Here's how the part is built. I have some questions about the finished solid (model axes, mm). A direction names the side the tool comes from. Give positions to 0.01 mm unless a question says otherwise; leave off trailing zeros. Loops run counter-clockwise (first coordinate to the right, second up) from the corner with the lowest first, then second, coordinate; pieces in that order, holes last.
Q1. Will these pins go through, and if not, where does the flat tip stop? P1, Ø8.5, axis at x = 6, y = -1, coming from the +Z side; P2, Ø24, axis at x = -3.5, y = 3, coming from the +Z side; P3, Ø6, axis at x = 0, y = 0, coming from the +Z side; P4, Ø1.2, axis at x = 0, y = 17, coming from the +Z side.
Q2. For faces 4 (the face through (0, -20, 2)), 5 (the face through (0, 24, 5)), which set-ups out of +Z, -Z, +X, -X, +Y, -Y let a thin tool reach every point of the face, with its end or its side?
Q3. If we section it at C-C (z = -2): Please give me the cut outline in (x, y), plus the area to 3 significant figures.
Q4. If we section it at D-D (y = -9.5): Please give me the cut outline in (x, z), plus the area to 3 significant figures.
Q5. We'd pull the mould along Z, two halves only. Please class faces 1 (the face through (0, 8, -5)), 2 (the face through (0, -6, 7)), 3 (the face through (0, 25, 2)): +Z half, -Z half, draft (parallel to the pull), parting line (faces both ways), or undercut.
Q6. I need wall thicknesses on line 1 (X direction, y = 0, z = 7.35); line 2 (Y direction, x = 0, z = 2.5); line 3 (Y direction, x = 0, z = 7.15). Which ranges of each line are inside material? Lowest first, please.
Q7. If we section it at B-B (z = 3.25): Give the number of separate pieces and of enclosed holes in the cut face, plus the area to 3 significant figures.
Q8. If we section it at A-A (y = 0): Please give me the cut outline in (x, z), plus the area to 3 significant figures.
from build123d import *

# Parameters (mm, degrees)
SKETCH_R          = 15
PAD_DEPTH         = 7
SKETCH001_R       = 2
PAD001_DEPTH      = 5
SKETCH002_R       = 15
SKETCH002_R_2     = 14
PAD002_DEPTH      = 7.4
SKETCH003_W       = 50
SKETCH003_H       = 45
PAD003_DEPTH      = 5
SKETCH004_W       = 50
SKETCH004_H       = 45
SKETCH004_W_2     = 48
SKETCH004_H_2     = 43
PAD004_DEPTH      = 10
SKETCH005_R       = 5
POCKET_DEPTH      = 5.001
POCKET_DEPTH_BACK = -10.001
SKETCH006_R       = 2
POCKET001_DEPTH   = 4


with BuildPart() as part:
    # Sketch → Pad (new body)
    with BuildSketch(Plane.XY):
        Circle(SKETCH_R)
    extrude(amount=PAD_DEPTH)

    # Sketch001 → Pad001 (join)
    with BuildSketch(Plane.XY):
        with BuildLine():
            add(Edge.make_bspline(
                [(-9.089263, 11.932531), (-7.058013, 18.679317), (0, 23.549677), (7.058013, 18.679317), (9.089263, 11.932531)],
                knots=[0, 0, 0, 0, 0.5, 1, 1, 1, 1], degree=3))
            Line((9.089263, 11.932531), (-9.089263, 11.932531))
        make_face()
        with Locations((0, 17.442505)):
            Circle(SKETCH001_R, mode=Mode.SUBTRACT)
    extrude(amount=PAD001_DEPTH)

    # Sketch002 → Pad002 (join)
    with BuildSketch(Plane.XY):
        Circle(SKETCH002_R)
        Circle(SKETCH002_R_2, mode=Mode.SUBTRACT)
    extrude(amount=PAD002_DEPTH)

    # Sketch003 → Pad003 (join)
    with BuildSketch(Plane.XY):
        with Locations((0, 2.5)):
            Rectangle(SKETCH003_W, SKETCH003_H)
    extrude(amount=-PAD003_DEPTH)

    # Sketch004 → Pad004 (join)
    with BuildSketch(Plane.XY):
        with Locations((0, 2.5)):
            Rectangle(SKETCH004_W, SKETCH004_H)
        with Locations((0, 2.5)):
            Rectangle(SKETCH004_W_2, SKETCH004_H_2, mode=Mode.SUBTRACT)
    extrude(amount=PAD004_DEPTH)

    # Sketch005 → Pocket (cut, two sides)
    with BuildSketch(Plane.XY) as pocket_sk:
        Circle(SKETCH005_R)
    extrude(amount=-POCKET_DEPTH, mode=Mode.SUBTRACT)
    extrude(pocket_sk.sketch, amount=-POCKET_DEPTH_BACK, mode=Mode.SUBTRACT)

    # Sketch006 → Pocket001 (cut)
    with BuildSketch(Plane.XY):
        with Locations((0, 17.442505)):
            Circle(SKETCH006_R)
    extrude(amount=-POCKET001_DEPTH, mode=Mode.SUBTRACT)


solid = part.part
Check sheet entries:
1. P1: stops at z = 7
1. P2: stops at z = 7.4
1. P3: passes through
1. P4: stops at z = -4
2. face 4: +Z, -Z, +X, -X, -Y
2. face 5: +Z
3. outline: (-25, -20) - (25, -20) - (25, 25) - (-25, 25) - close; hole circle Ø10 at (0, 0); hole circle Ø4 at (0, 17.44)
3. area: 2,160 mm2
4. outline: (-25, -5) - (25, -5) - (25, 10) - (24, 10) - (24, 0) - (11.61, 0) - (11.61, 7.4) - (10.28, 7.4) - (10.28, 7) - (-10.28, 7) - (-10.28, 7.4) - (-11.61, 7.4) - (-11.61, 0) - (-24, 0) - (-24, 10) - (-25, 10) - close
4. area: 434 mm2
5. face 1: -Z half
5. face 2: +Z half
5. face 3: draft
6. line 1: x = -25 to -24, -15 to -14, 14 to 15, 24 to 25
6. line 2: y = -20 to -19, -15 to -5, 5 to 15.44, 19.44 to 21.11, 24 to 25
6. line 3: y = -20 to -19, -15 to -14, 14 to 15, 24 to 25
7. separate pieces: 2
7. enclosed holes: 3
7. area: 885 mm2
8. outline: (-25, -5) - (-5, -5) - (-5, 7) - (-14, 7) - (-14, 7.4) - (-15, 7.4) - (-15, 0) - (-24, 0) - (-24, 10) - (-25, 10) - close; (5, -5) - (25, -5) - (25, 10) - (24, 10) - (24, 0) - (15, 0) - (15, 7.4) - (14, 7.4) - (14, 7) - (5, 7) - close
8. area: 361 mm2
